Drawing for the job (mm, zero at the part's lowest x, y, z). A direction names the side the tool comes from. Give positions to 0.01 mm unless a question says otherwise; leave off trailing zeros. Loops run counter-clockwise (first coordinate to the right, second up) from the corner with the lowest first, then second, coordinate; pieces in that order, holes last.
1) Band-saw the part on C-C on x = 65. List the corners of the cut face in (y, z).
2) Band-saw the part on B-B on x = 18. List the corners of the cut face in (y, z).
3) 3-axis set-ups, long thin cutter, end or side, ignore diameter. For the marked faces 1, 2, 3 and 4: which of +Z, -Z, +X, -X, +Y, -Y reach the whole face in a straight line?
4) Wall check: line 1 (X direction, y = 25, z = 29); line 2 (Z direction, x = 91, y = 28.5); line 3 (Z direction, x = 8, y = 21.5). Give the ranges that are in metal, low to high.
5) Two-plate mould, pull along Z, no slides. Class the marked faces 5, 6 and 7: +Z half, -Z half, draft (parallel to the pull), parting line (faces both ways), or undercut.
6) Band-saw the part on A-A on z = 34.5. List the corners of the cut face in (x, y).
7) Band-saw the part on D-D on y = 47. List the corners of the cut face in (x, z), then the cut area to 3 significant figures.
8) Flat gauge pins, fed straight in: P1, Ø6.5, axis at x = 58.5, y = 39.5, coming from the -Z side; P2, Ø4, axis at y = 24.5, z = 45, coming from the +X side. Where does each tip first touch, or does it go through?
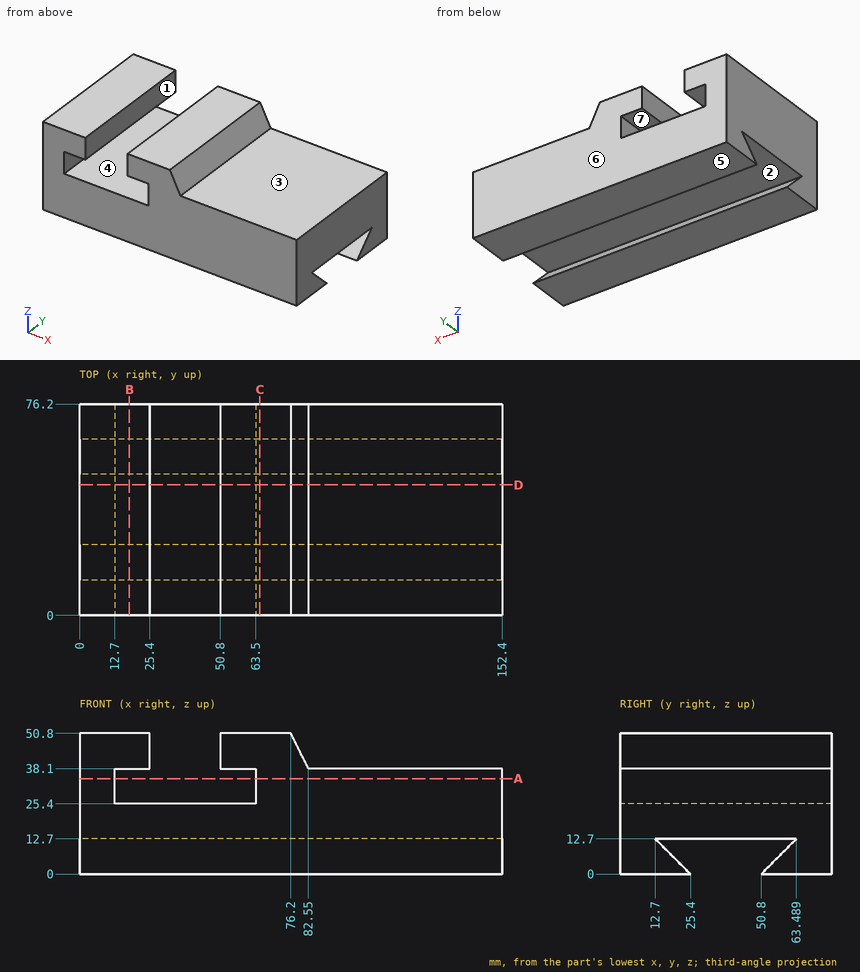
Findings below:
1. outline: (0, 0) - (25.4, 0) - (12.7, 12.7) - (63.49, 12.7) - (50.8, 0) - (76.2, 0) - (76.2, 50.8) - (0, 50.8) - close
2. outline: (0, 0) - (25.4, 0) - (12.7, 12.7) - (63.49, 12.7) - (50.8, 0) - (76.2, 0) - (76.2, 25.4) - (0, 25.4) - close; (0, 38.1) - (76.2, 38.1) - (76.2, 50.8) - (0, 50.8) - close
3. face 1: +Z, +Y, -Y
3. face 2: +X, -X
3. face 3: +Z, +X, +Y, -Y
3. face 4: +Y, -Y
4. line 1: x = 0 to 12.7, 63.5 to 152.4
4. line 2: z = 12.7 to 38.1
4. line 3: z = 0 to 3.9, 12.7 to 50.8
5. face 5: -Z half
5. face 6: draft
5. face 7: undercut
6. outline: (0, 0) - (12.7, 0) - (12.7, 76.2) - (0, 76.2) - close; (63.5, 0) - (152.4, 0) - (152.4, 76.2) - (63.5, 76.2) - close
7. outline: (0, 12.7) - (152.4, 12.7) - (152.4, 38.1) - (82.55, 38.1) - (76.2, 50.8) - (50.8, 50.8) - (50.8, 38.1) - (63.5, 38.1) - (63.5, 25.4) - (12.7, 25.4) - (12.7, 38.1) - (25.4, 38.1) - (25.4, 50.8) - (0, 50.8) - close
7. area: 3,910 mm2
8. P1: stops at z = 12.7
8. P2: stops at x = 80.1
